```python
from build123d import *

# Parameters (mm, degrees)
ESBO_O1_R                = 4
RESSALTO_EXTRUS_O1_DEPTH = 10
ESBO_O2_R                = 1
CORTE_EXTRUS_O1_DEPTH    = 10
ESBO_O3_R                = 1
CORTE_EXTRUS_O2_DEPTH    = 20
ESBO_O5_R                = 3
CORTE_EXTRUS_O3_DEPTH    = 6


with BuildPart() as part:
    # Esboço1 → Ressalto-extrusão1 (new body)
    with BuildSketch(Plane.XY):
        with BuildLine():
            Line((-23.5, 0), (-23.5, 12.766875201))
            ThreePointArc((-23.5, 12.766875201), (-22.035533906, 16.302409107), (-18.5, 17.766875201))
            Line((-18.5, 17.766875201), (18.5, 17.766875201))
            ThreePointArc((18.5, 17.766875201), (22.035533906, 16.302409107), (23.5, 12.766875201))
            Line((23.5, 12.766875201), (23.5, 0))
            ThreePointArc((23.5, 0), (21.449747468, -4.949747468), (16.5, -7))
            Line((16.5, -7), (7.047816286, -7))
            Line((7.047816286, -7), (7.047816286, 8))
            Line((7.047816286, 8), (4.047816286, 8))
            Line((4.047816286, 8), (4.047816286, -7))
            Line((4.047816286, -7), (2.547816286, -7))
            Line((2.547816286, -7), (2.547816286, 8))
            Line((2.547816286, 8), (-8.5, 8))
            Line((-8.5, 8), (-9.5, 0))
            ThreePointArc((-9.5, 0), (-16.5, -7), (-23.5, 0))
        make_face()
        with Locations((-16.5, 0)):
            Circle(ESBO_O1_R, mode=Mode.SUBTRACT)
        with Locations((16.5, 0)):
            Circle(ESBO_O1_R, mode=Mode.SUBTRACT)
    extrude(amount=RESSALTO_EXTRUS_O1_DEPTH)

    # Esboço2 → Corte-extrusão1 (cut, along a direction that is not the sketch's normal)
    with BuildSketch(Plane.ZY.offset(-2.547816286)):
        with Locations((5, -5.228639013)):
            Circle(ESBO_O2_R)
    extrude(amount=-CORTE_EXTRUS_O1_DEPTH, dir=(-0.931482298, -0.363786654, 0), mode=Mode.SUBTRACT)

    # Esboço3 → Corte-extrusão2 (cut)
    with BuildSketch(Plane(origin=(0, 17.766875201, 0), x_dir=(1, 0, 0), z_dir=(0, 1, 0))):
        with Locations((-16.5, -5)):
            Circle(ESBO_O3_R)
        with Locations((16.5, -5)):
            Circle(ESBO_O3_R)
    extrude(amount=-CORTE_EXTRUS_O2_DEPTH, mode=Mode.SUBTRACT)

    # Esboço5 → Corte-extrusão3 (cut)
    with BuildSketch(Plane(origin=(0, 17.766875201, 0), x_dir=(1, 0, 0), z_dir=(0, 1, 0))):
        with Locations((-16.5, -5)):
            Circle(ESBO_O5_R)
        with Locations((16.5, -5)):
            Circle(ESBO_O5_R)
    extrude(amount=-CORTE_EXTRUS_O3_DEPTH, mode=Mode.SUBTRACT)


solid = part.part
```
Model file for the job. Use its own axes, mm. A direction names the side the tool comes from. Coordinates: 2 decimals unless noted, no trailing zeros. Write each loop counter-clockwise with the first axis right and the second up, starting at its lowest first coordinate (ties: lowest second). Pieces come first, ordered by that corner, then holes. Notation, with made-up numbers: (80.25, 20) - (112.25, 20) arc R23 ccw to (112.25, 56) - close; hole circle Ø3 at (69.25, -3). An arc over 180 degrees is marked (long way). Use a Markdown table: item, result. Add a question column.
Item 1: Band-saw the part on A-A, the plane x = -16.5. Write the cut outline in (y, z), and give its area (3 significant figures).
Item 2: Band-saw the part on B-B, the plane y = 2.75. Write the cut outline in (x, z), and give its area (3 significant figures).
Item 3: Band-saw the part on D-D, the plane x = 19. Write the cut outline in (y, z).
Item 4: 3-axis set-ups, long thin cutter, end or side, ignore diameter. For faces 1 (the face through (3, -7, 5)), 2 (the face through (18, 11.767, 5)), 3 (the face through (6, 8, 5)): which of +Z, -Z, +X, -X, +Y, -Y reach the whole face in a straight line?
Item 5: Drill centre lines: line 1 along Y through (x, z) = (-16.5, 7.75); line 2 along X through (y, z) = (16.5, 7.25); line 3 along X through (y, z) = (-2.5, 7). Where is each one in solid material? Low to high.
Item 6: Two-plate mould, pull along Y, no slides. Class faces 4 (the face through (11.863, -2, 5)), 5 (the face through (0.3, 8.3, 10)), 6 (the face through (0, 17.767, 5)): pulls with the +Y half, pulls with the -Y half, needs draft (parallel to the pull), parting line crosses it, or undercut.
Item 7: Drop flat-ended pins along their axis: pin 1 (3.5 mm diameter, centred on x = 16.5, z = 5, fed in from +Y); pin 2 (0.9 mm diameter, centred on x = 6, z = 3.5, fed in from -Y); pin 3 (1.6 mm diameter, centred on y = -1.5, z = 5.5, fed in from -X). Give the stop position or say it passes through.
Item 8: Band-saw the part on C-C, the plane z = 1.5. Write the cut outline in (x, y).
A:
| question | item | result |
|---|---|---|
| 1 | outline | (-7, 0) - (-4, 0) - (-4, 10) - (-7, 10) - close; (4, 0) - (17.77, 0) - (17.77, 2) - (11.77, 2) - (11.77, 4) - (4, 4) - close; (4, 6) - (11.77, 6) - (11.77, 8) - (17.77, 8) - (17.77, 10) - (4, 10) - close |
| 1 | area | 116 mm² |
| 2 | outline | (-23.5, 0) - (-19.4, 0) - (-19.4, 10) - (-23.5, 10) - close; (-13.6, 0) - (-9.16, 0) - (-9.16, 10) - (-13.6, 10) - close; (2.55, 0) - (4.05, 0) - (4.05, 10) - (2.55, 10) - close; (7.05, 0) - (13.6, 0) - (13.6, 10) - (7.05, 10) - close; (19.4, 0) - (23.5, 0) - (23.5, 10) - (19.4, 10) - close |
| 2 | area | 207 mm² |
| 3 | outline | (-6.54, 0) - (-3.12, 0) - (-3.12, 10) - (-6.54, 10) - close; (3.12, 0) - (17.74, 0) - (17.74, 3.34) - (11.77, 3.34) - (11.77, 6.66) - (17.74, 6.66) - (17.74, 10) - (3.12, 10) - close |
| 4 | face 1 | +Z, -Z, +X, -X, -Y |
| 4 | face 2 | +Y |
| 4 | face 3 | +Z, -Z, -Y |
| 5 | line 1 | y = -7 to -4, 4 to 11.77 |
| 5 | line 2 | x = -21.83 to -18.48, -14.52 to 14.52, 18.48 to 21.83 |
| 5 | line 3 | x = -23.04 to -19.62, -13.38 to -9.96, 2.55 to 4.05, 7.05 to 13.38, 19.62 to 23.04 |
| 6 | face 4 | undercut |
| 6 | face 5 | needs draft |
| 6 | face 6 | pulls with the +Y half |
| 7 | pin 1 | stops at y = 11.77 |
| 7 | pin 2 | stops at y = 8 |
| 7 | pin 3 | stops at x = -23.46 |
| 8 | outline | (-23.5, 0) arc R7 ccw to (-9.5, 0) - (-8.5, 8) - (2.55, 8) - (2.55, -7) - (4.05, -7) - (4.05, 8) - (7.05, 8) - (7.05, -7) - (16.5, -7) arc R7 ccw to (23.5, 0) - (23.5, 12.77) arc R5 ccw to (18.5, 17.77) - (-18.5, 17.77) arc R5 ccw to (-23.5, 12.77) - close; hole circle Ø8 at (-16.5, 0); hole circle Ø8 at (16.5, 0) |
